```python
from build123d import *

# Parameters (mm, degrees)
SKETCH_1_W                = 37
SKETCH_1_H                = 7
EXTRUDE_1_DEPTH           = 1
SKETCH_3_W                = 30.866999712
SKETCH_3_H                = 13
EXTRUDE_2_DEPTH           = 7
SKETCH_4_W                = 30.866999712
SKETCH_4_H                = 8
EXTRUDE_3_DEPTH           = 11
SKETCH_5_W                = 14.630132385
SKETCH_5_H                = 6.854419706
SKETCH_5_W_2              = 7.444047208
EXTRUDE_4_DEPTH           = 13.2
SKETCH_6_R                = 3.5
EXTRUDE_5_DEPTH           = 1
HOLE_WIZARD_3_0_3_1_D     = 3
HOLE_WIZARD_3_0_3_1_DEPTH = 8.5
HOLE_WIZARD_3_0_3_1_TIP   = 0.901290929


with BuildPart() as part:
    # 草图1 → 凸台-拉伸1 (new body)
    with BuildSketch(Plane.XY):
        Rectangle(SKETCH_1_W, SKETCH_1_H)
    extrude(amount=EXTRUDE_1_DEPTH)

    # 草图3 → 凸台-拉伸2 (add)
    with BuildSketch(Plane.XY):
        Rectangle(SKETCH_3_W, SKETCH_3_H)
    extrude(amount=EXTRUDE_2_DEPTH)

    # 草图4 → 凸台-拉伸3 (add)
    with BuildSketch(Plane.XY):
        Rectangle(SKETCH_4_W, SKETCH_4_H)
    extrude(amount=EXTRUDE_3_DEPTH)

    # 草图5 → 凸台-拉伸4 (add)
    with BuildSketch(Plane.XY):
        with Locations((-7.315066193, 0)):
            Rectangle(SKETCH_5_W, SKETCH_5_H)
        with Locations((9.360336589, 0)):
            Rectangle(SKETCH_5_W_2, SKETCH_5_H)
    extrude(amount=EXTRUDE_4_DEPTH)

    # 草图6 → 凸台-拉伸5 (add)
    with BuildSketch(Plane.XY.offset(1)):
        with Locations((18.5, 0)):
            Circle(SKETCH_6_R)
        with Locations((-18.5, 0)):
            Circle(SKETCH_6_R)
    extrude(amount=-EXTRUDE_5_DEPTH)

    # Ø3.0 (3) 直径孔1
    with Locations(Plane.XY.offset(1)):
        with Locations((-18.5, 0), (18.5, 0)):
            Hole(HOLE_WIZARD_3_0_3_1_D / 2, depth=HOLE_WIZARD_3_0_3_1_DEPTH)
            with Locations((0, 0, -(HOLE_WIZARD_3_0_3_1_DEPTH + HOLE_WIZARD_3_0_3_1_TIP / 2))):  # 118° drill point
                Cone(0, HOLE_WIZARD_3_0_3_1_D / 2, HOLE_WIZARD_3_0_3_1_TIP, mode=Mode.SUBTRACT)


solid = part.part
```
For this review, take the finished solid that the model builds, in its own axes (mm). A direction names the side the tool comes from. Round coordinates to 2 decimals unless told otherwise and drop trailing zeros. Write each loop counter-clockwise with the first axis right and the second up, starting at its lowest first coordinate (ties: lowest second). Pieces come first, ordered by that corner, then holes.
1) Take a section at C-C on z = 1.5. Give the boundary of the cut face in (x, y).
Answer below:
outline: (-15.43, -6.5) - (15.43, -6.5) - (15.43, 6.5) - (-15.43, 6.5) - close
2) Take a section at B-B on x = 7.5. Give the boundary of the cut face in (y, z), then the cut area to 3 significant figures.
Answer below:
outline: (-6.5, 0) - (6.5, 0) - (6.5, 7) - (4, 7) - (4, 11) - (3.43, 11) - (3.43, 13.2) - (-3.43, 13.2) - (-3.43, 11) - (-4, 11) - (-4, 7) - (-6.5, 7) - close
area: 138 mm2
3) Take a section at A-A on y = 0. Give the boundary of the cut face in (x, z).
Answer below:
outline: (-22, 0) - (-20, 0) - (-20, 1) - (-22, 1) - close; (-17, 0) - (17, 0) - (17, 1) - (15.43, 1) - (15.43, 11) - (13.08, 11) - (13.08, 13.2) - (5.64, 13.2) - (5.64, 11) - (0, 11) - (0, 13.2) - (-14.63, 13.2) - (-14.63, 11) - (-15.43, 11) - (-15.43, 1) - (-17, 1) - close; (20, 0) - (22, 0) - (22, 1) - (20, 1) - close
4) Take a section at D-D on y = 5.25. Give the boundary of the cut face in (x, z), then the cut area to 3 significant figures.
Answer below:
outline: (-15.43, 0) - (15.43, 0) - (15.43, 7) - (-15.43, 7) - close
area: 216 mm2
5) For line 1 along Y through (x, z) = (18.5, 0.6); line 2 along X through (y, z) = (0.75, 12.75); line 3 along X through (y, z) = (4.25, 3), list the stretches that pass through material, from the lowest coordinate up.
Answer below:
line 1: y = -3.5 to -1.5, 1.5 to 3.5
line 2: x = -14.63 to 0, 5.64 to 13.08
line 3: x = -15.43 to 15.43
6) Mouldability with a two-part tool opening along X and no side actions: class faces 4 (the face through (-22, 0.1, 0.5)), 5 (the face through (-17, 0.07, 0.49)), 6 (the face through (16.9, 3.5, 0.5)) as +X half, -X half, draft (parallel to the pull), parting line (faces both ways), or undercut.
Answer below:
face 4: -X half
face 5: undercut
face 6: draft
7) Machinability: for faces 1 (the face through (16.9, -3.5, 0.5)), 2 (the face through (0, 4, 9)), 3 (the face through (9, -3.427, 12)), which of the approach directions +Z, -Z, +X, -X, +Y, -Y give a long, thin tool a straight path to every point of the face, cutting with its end or side? Answer none if there is none.
Answer below:
face 1: +Z, -Z, +X, -Y
face 2: +Z, +X, -X, +Y
face 3: +Z, +X, -X, -Y
8) Insertion check: pin 1 Ø7 at (x, y) = (-19, -1) entering from +Z; pin 2 Ø2.5 at (y, z) = (1, 11.5) entering from -X; pin 3 Ø0.8 at (x, z) = (17.5, 0.5) entering from +Y; pin 4 Ø1.8 at (x, y) = (18.5, 0) entering from +Z. Each pin has a flat end and moves straight along its axis. Give the tip position at first contact, or say it passes through.
Answer below:
pin 1: stops at z = 1
pin 2: stops at x = -15.43
pin 3: stops at y = 3.5
pin 4: passes through
